Source: three-view drawing plus pictorial views. Frame: mm from the lowest corner of the part. Give positions to 0.01 mm unless a question says otherwise; leave off trailing zeros. Write each loop counter-clockwise with the first axis right and the second up, starting at its lowest first coordinate (ties: lowest second). Pieces come first, ordered by that corner, then holes. Notation, with made-up numbers: (-24, 41) -> (33, 41) arc R24 cw to (33, 59) -> close; hole circle Ø9 at (75.25, -29). An arc over 180 degrees is marked (long way). Write item = value, one per line.
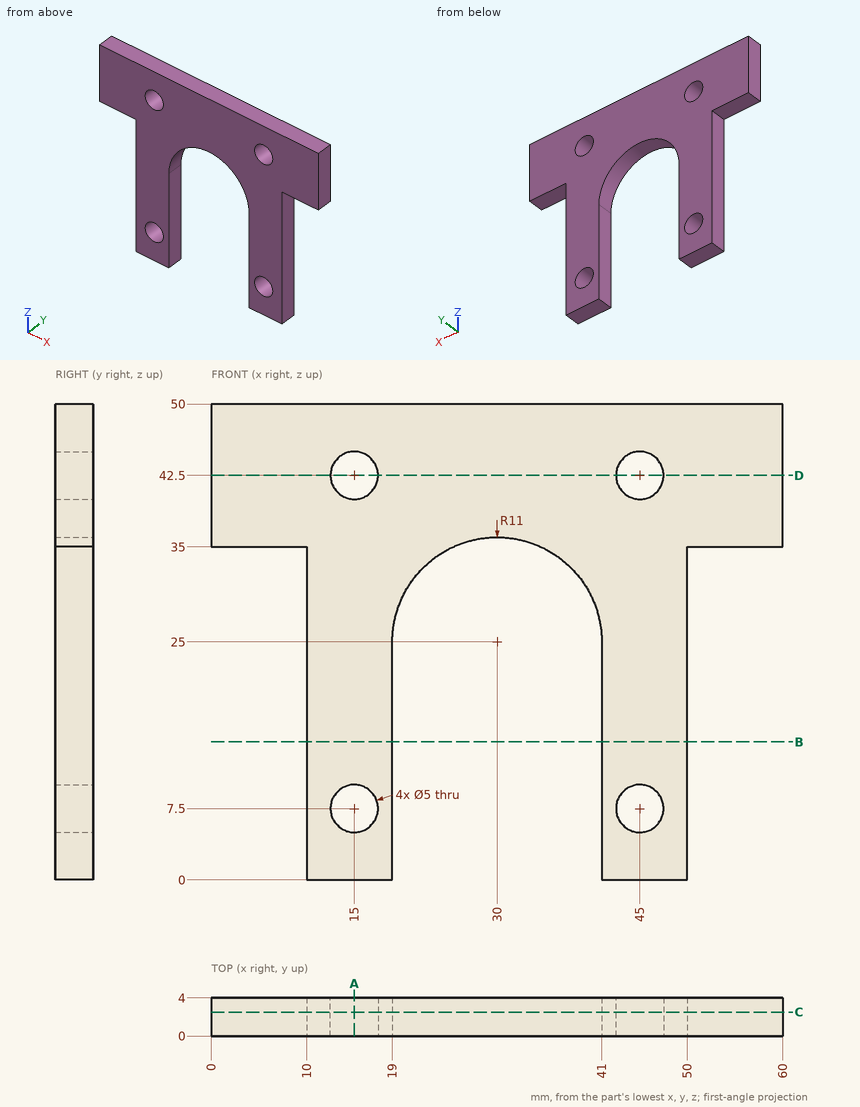
1) Contact query for flat-ended pins moving along their axis: pin 1 (2 mm diameter, centred on y = 1.5, z = 12.5, fed in from -X); pin 2 (2 mm diameter, centred on y = 2, z = 15.5, fed in from +X); pin 3 (1.2 mm diameter, centred on x = 54, y = 3, fed in from -Z). Output: stop coordinate, or through.
Computed:
pin_1 = 10
pin_2 = 50
pin_3 = 35
2) Cut plane D-D (z = 42.5). Return the cut outline in (x, y).
Computed:
outline = (0, 0) -> (12.5, 0) -> (12.5, 4) -> (0, 4) -> close; (17.5, 0) -> (42.5, 0) -> (42.5, 4) -> (17.5, 4) -> close; (47.5, 0) -> (60, 0) -> (60, 4) -> (47.5, 4) -> close
3) Cut plane A-A (x = 15). Return the cut outline in (y, z), then the cut area to 3 significant figures.
Computed:
outline = (0, 0) -> (4, 0) -> (4, 5) -> (0, 5) -> close; (0, 10) -> (4, 10) -> (4, 40) -> (0, 40) -> close; (0, 45) -> (4, 45) -> (4, 50) -> (0, 50) -> close
area = 160 mm²
4) Cut plane C-C (y = 2.5). Return the cut outline in (x, z), then the cut area to 3 significant figures.
Computed:
outline = (0, 35) -> (10, 35) -> (10, 0) -> (19, 0) -> (19, 25) arc R11 cw to (41, 25) -> (41, 0) -> (50, 0) -> (50, 35) -> (60, 35) -> (60, 50) -> (0, 50) -> close; hole circle Ø5 at (15, 7.5); hole circle Ø5 at (15, 42.5); hole circle Ø5 at (45, 7.5); hole circle Ø5 at (45, 42.5)
area = 1,480 mm²
5) Material intervals for L1, parallel to Z at x = 45, y = 1.9; L2, parallel to X at y = 0.8, z = 16.5; L3, parallel to Z at x = 14, y = 0.65, sorted ascending.
Computed:
L1 = 0 to 5, 10 to 40, 45 to 50
L2 = 10 to 19, 41 to 50
L3 = 0 to 5.21, 9.79 to 40.21, 44.79 to 50
6) Cut plane B-B (z = 14.5). Return the cut outline in (x, y).
Computed:
outline = (10, 0) -> (19, 0) -> (19, 4) -> (10, 4) -> close; (41, 0) -> (50, 0) -> (50, 4) -> (41, 4) -> close
